Check sheet for the modelled part. Datum: model origin and axes. Units: mm. A direction names the side the tool comes from. Give positions to 0.01 mm unless a question says otherwise; leave off trailing zeros. Loops run counter-clockwise (first coordinate to the right, second up) from the corner with the lowest first, then second, coordinate; pieces in that order, holes last. Notation, with made-up numbers: (63, -38.5) - (113, -38.5) arc R23 cw to (113, -0.5) - close; hole circle Ø9 at (-0.75, -8). An arc over 180 degrees is marked (long way). Answer in a Markdown table with one row per item. Add a question column.
(1) Go/stop test with flat-tipped pins: P1, Ø2, axis at x = 41.5, z = 3, coming from the -Y side; P2, Ø1.5, axis at x = 70.5, y = 0, coming from the +Z side; P3, Ø3, axis at x = 63, z = -3, coming from the -Y side; P4, Ø4, axis at x = 11.5, y = 1.5, coming from the -Z side. Record where each tip stops, or that it passes through.
(2) Set-up check for faces 4 (the face through (6, 2, 0)), 5 (the face through (104, 0, 0)), 6 (the face through (99, 2, 0)): record each of +Z, -Z, +X, -X, +Y, -Y from which the full face is reachable in a straight line by a thin tool's end or side.
(3) Sectioned sample at C-C on x = 91. Enter the section's corners in (y, z).
(4) Thickness scan on L1, parallel to X at y = 3, z = -1; L2, parallel to Z at x = 67, y = -2.25; L3, parallel to X at y = -2.75, z = -0.5. Record the ranges inside material, lowest first.
(5) Draft check along X on faces 1 (the face through (94, -2, -1)), 2 (the face through (51.44, -0.9, 2.86)), 3 (the face through (0, 0, 0)). Enter one of: released by +X, released by -X, zero draft, split by the parting line, or undercut.
from build123d import *

# Parameters (mm, degrees)
SKETCH2_W           = 10
SKETCH2_H           = 2
SKETCH3_R           = 4
BOSS_EXTRUDE1_DEPTH = 2
FILLET1_R           = 1
CHAMFER1_SIZE       = 1
CHAMFER2_SIZE       = 1
BOSS_EXTRUDE2_START = -2
SKETCH4_R           = 4
BOSS_EXTRUDE2_DEPTH = 2
FILLET2_R           = 1


with BuildPart() as part:
    # Sketch2 → Revolve2 (revolve)
    with BuildSketch(Plane.XY, mode=Mode.PRIVATE) as revolve2_sk:
        with Locations((99, 1)):
            Rectangle(SKETCH2_W, SKETCH2_H)
        Polygon((10, 2), (10, 0), (94, 0), (94, 2), (94, 3), (10, 3), align=None)
        with Locations((5, 1)):
            Rectangle(SKETCH2_W, SKETCH2_H)
    revolve(revolve2_sk.sketch.rotate(Axis((0, 0, 0), (1, 0, 0)), 90), axis=Axis((0, 0, 0), (1, 0, 0)))

    # Sketch3 → Boss-Extrude1 (add)
    with BuildSketch(Plane(origin=(94, 0, 0), x_dir=(0, 0, -1), z_dir=(1, 0, 0))):
        Circle(SKETCH3_R)
    extrude(amount=-BOSS_EXTRUDE1_DEPTH)

    # Fillet1
    fillet1_edges = [part.edges().sort_by_distance(p)[0] for p in [
        (92, 0, 4),
        (94, 0, 4),
    ]]
    fillet(fillet1_edges, radius=FILLET1_R - 0.0001)  # a hair under: the kernel refuses the full size

    # Chamfer1
    chamfer1_edges = [part.edges().sort_by_distance(p)[0] for p in [
        (104, 0, -2),
    ]]
    chamfer(chamfer1_edges, length=CHAMFER1_SIZE)

    # Chamfer2
    chamfer2_edges = [part.edges().sort_by_distance(p)[0] for p in [
        (0, 0, -2),
    ]]
    chamfer(chamfer2_edges, length=CHAMFER2_SIZE)

    # Sketch4 → Boss-Extrude2 (add)
    with BuildSketch(Plane.ZY.offset(-10).offset(BOSS_EXTRUDE2_START)):
        Circle(SKETCH4_R)
    extrude(amount=BOSS_EXTRUDE2_DEPTH)

    # Fillet2
    fillet2_edges = [part.edges().sort_by_distance(p)[0] for p in [
        (12, 0, -4),
        (10, 0, -4),
    ]]
    fillet(fillet2_edges, radius=FILLET2_R - 0.0001)  # a hair under: the kernel refuses the full size


solid = part.part
Reply:
| question | item | result |
|---|---|---|
| 1 | P1 | y = -2.24 |
| 1 | P2 | z = 3 |
| 1 | P3 | y = -2.6 |
| 1 | P4 | z = -4 |
| 2 | face 4 | -X |
| 2 | face 5 | +Z, -Z, +X, +Y, -Y |
| 2 | face 6 | +X |
| 3 | outline | circle Ø6 at (0, 0) |
| 4 | L1 | 10.01 to 11.99, 92.01 to 93.99 |
| 4 | L2 | -1.98 to 1.98 |
| 4 | L3 | 10 to 94 |
| 5 | face 1 | released by +X |
| 5 | face 2 | undercut |
| 5 | face 3 | released by -X |
